Could you check a few things on this model? Use its own coordinates, in mm. A direction names the side the tool comes from. Round coordinates to 2 decimals unless told otherwise and drop trailing zeros. Order: outer loops, then holes, each group sorted by start corner. A loop starts at its lowest first (then second) coordinate and runs counter-clockwise, first axis right, second up. Notation, with made-up numbers: (58.5, 50) -> (114.5, 50) arc R32 ccw to (114.5, 77) -> close; hole circle Ø4 at (58.5, 60). An arc over 180 degrees is marked (long way). One line per question, with ' | ' between items.
```python
from build123d import *

# Parameters (mm, degrees)
F0_W      = 22
F0_H      = 17.78
F1_DEPTH  = 6.35
F2_W      = 3.7016793489
F2_H      = 17.78
F3_DEPTH  = 39
F6_R      = 2.5527
F8_DEPTH  = 25
F4_R      = 3.2512
F7_R      = 1.524
F10_R     = 1.778
F11_DEPTH = 25
F12_R     = 1.778
F13_DEPTH = 2.54
F14_R     = 5
F15_R     = 0.5


with BuildPart() as f1:
    # F0 (on Top) → F1 (new body)
    with BuildSketch(Plane.XY):
        Rectangle(F0_W, F0_H)
    extrude(amount=F1_DEPTH)

    # F2 (on Top) → F3 (join)
    with BuildSketch(Plane.XY):
        with Locations((-12.8508396745, 0)):
            Rectangle(F2_W, F2_H)
    extrude(amount=F3_DEPTH)

    # F6 (on Top) → F8 (cut)
    with BuildSketch(Plane.XY):
        Circle(F6_R)
    extrude(amount=F8_DEPTH, mode=Mode.SUBTRACT)

    # F4 (on face) → F9 section 0
    with BuildSketch(Plane.XY.offset(6.35)):
        Circle(F4_R)
    # F7 (on offset) → F9 section 1
    with BuildSketch(Plane.XY.offset(3.8862)):
        Circle(F7_R)
    loft(mode=Mode.SUBTRACT)

    # F10 (on face) → F11 (cut)
    with BuildSketch(Plane.YZ.offset(-11)):
        with Locations((0, 33.75)):
            Circle(F10_R)
    extrude(amount=-F11_DEPTH, mode=Mode.SUBTRACT)

    # F12 (on face) → F13 (cut)
    with BuildSketch(Plane(origin=(-14.7016793489, 0, 0), x_dir=(0, -1, 0), z_dir=(-1, 0, 0))):
        Polygon((3.5062095774, 30.91573349), (4.2076515874, 35.36933331), (0.7014420101, 38.20359982), (-3.5062095774, 36.58426651), (-4.2076515874, 32.13066669), (-0.7014420101, 29.29640018), align=None)
        with Locations((0, 33.75)):
            Circle(F12_R, mode=Mode.SUBTRACT)
    extrude(amount=-F13_DEPTH, mode=Mode.SUBTRACT)

    # F14
    f14_edges = [f1.edges().sort_by_distance(p)[0] for p in [
        (11, 8.89, 3.175),
        (11, -8.89, 3.175),
        (-12.85084, 8.89, 39),
        (-12.85084, -8.89, 39),
    ]]
    fillet(f14_edges, radius=F14_R)

    # F15
    f15_edges = [f1.edges().sort_by_distance(p)[0] for p in [
        (-11, -8.89, 20.175),
        (-11, 0, 6.35),
        (-14.701679, -8.89, 17),
        (-14.701679, -7.425534, 37.535534),
        (11, 0, 6.35),
        (9.535534, -7.425534, 6.35),
        (9.535534, 7.425534, 6.35),
        (-2.5, -8.89, 6.35),
        (-2.5, 8.89, 6.35),
        (-11, 8.89, 20.175),
        (-14.701679, 8.89, 17),
        (-14.701679, 7.425534, 37.535534),
        (-14.701679, 0, 39),
        (-11, 7.425534, 37.535534),
        (-11, 0, 39),
        (-11, -7.425534, 37.535534),
    ]]
    fillet(f15_edges, radius=F15_R)


solid = f1.part
```
1. I want a section at D-D on y = 0. Count the separate pieces of the cut face and the enclosed holes in it, and give its area (3 significant figures).
From the geometry:
separate pieces: 3 | enclosed holes: 0 | area: 225 mm²
2. I want a section at B-B on z = 26.5. List the corners of the cut face in (x, y) for me, and give its area (3 significant figures).
From the geometry:
outline: (-14.7, -8.39) arc R0.5 ccw to (-14.2, -8.89) -> (-11.5, -8.89) arc R0.5 ccw to (-11, -8.39) -> (-11, 8.39) arc R0.5 ccw to (-11.5, 8.89) -> (-14.2, 8.89) arc R0.5 ccw to (-14.7, 8.39) -> close | area: 65.6 mm²
3. I want a section at C-C on x = -5.75. List the corners of the cut face in (y, z) for me.
From the geometry:
outline: (-8.89, 0) -> (8.89, 0) -> (8.89, 5.85) arc R0.5 ccw to (8.39, 6.35) -> (-8.39, 6.35) arc R0.5 ccw to (-8.89, 5.85) -> close
4. I'm going to push flat-ended pins straight in: pin 1 (5 mm diameter, centred on y = 2, z = 18.5, fed in from +X); pin 2 (1.5 mm diameter, centred on x = -10, y = 4, fed in from +Z); pin 3 (10 mm diameter, centred on x = 3.5, y = -1, fed in from +Z). Where does each tip first touch, or does it pass through?
From the geometry:
pin 1: stops at x = -11 | pin 2: stops at z = 6.42 | pin 3: stops at z = 6.35
5. I need wall thicknesses on probe 1 along Y at (x, z) = (0, 2.9); probe 2 along Y at (x, z) = (-11.85, 33.75); probe 3 along X at (y, z) = (0, 2.7). Which ranges of each line are inside material? Lowest first, please.
From the geometry:
probe 1: y = -8.89 to -2.55, 2.55 to 8.89 | probe 2: y = -8.89 to -1.78, 1.78 to 8.89 | probe 3: x = -14.7 to -2.55, 2.55 to 11
6. On a 3-axis mill with a long thin cutter (end or side, diameter ignored), from which of +Z, -Z, +X, -X, +Y, -Y can I reach the whole of each face in a straight line? I mean faces 4 (the face through (-11, 0, 22)), 5 (the face through (-12.162, -2, 34)), 6 (the face through (-11.573, -0.231, 35.513)). Say none if no direction works.
From the geometry:
face 4: +Z, +X, +Y, -Y | face 5: -X | face 6: +X, -X
7. I want a section at A-A on x = 0. List the corners of the cut face in (y, z) for me, and give its area (3 significant figures).
From the geometry:
outline: (-8.89, 0) -> (-2.55, 0) -> (-2.55, 5.35) -> (-3.25, 6.35) -> (-8.39, 6.35) arc R0.5 ccw to (-8.89, 5.85) -> close; (2.55, 0) -> (8.89, 0) -> (8.89, 5.85) arc R0.5 ccw to (8.39, 6.35) -> (3.25, 6.35) -> (2.55, 5.35) -> close | area: 79.7 mm²
8. If we mould it in two halves opening along Y, with no side actions, what happens to faces 1 (the face through (-12.83, -7.39, 37.57)), 2 (the face through (-12, 8.89, 11)), 3 (the face through (-13.45, -3.85, 33.11))? For each: pulls with the +Y half, pulls with the -Y half, needs draft (parallel to the pull), parting line crosses it, or undercut.
From the geometry:
face 1: pulls with the -Y half | face 2: pulls with the +Y half | face 3: undercut
